```python
from build123d import *

# Parameters (mm, degrees)
CROQUIS1_R                 = 15
SALIENTE_EXTRUIR1_DEPTH    = 175
CROQUIS2_R                 = 4.5
CORTAR_EXTRUIR1_DEPTH      = 177.281025638
CORTAR_EXTRUIR2_START      = 15
CORTAR_EXTRUIR2_DEPTH      = 4
CROQUIS4_R                 = 10
CORTAR_EXTRUIR3_DEPTH      = 177.281025756
CORTAR_EXTRUIR4_DEPTH      = 177.281025756
CORTAR_EXTRUIR4_DEPTH_BACK = 177.281025756
CROQUIS9_R                 = 4.5
CORTAR_EXTRUIR5_START      = 15
CORTAR_EXTRUIR5_DEPTH      = 4
CORTAR_EXTRUIR6_DEPTH      = 177.281025756
CORTAR_EXTRUIR6_DEPTH_BACK = 177.281025756
SALIENTE_EXTRUIR2_START    = 30
CROQUIS16_R                = 17
CROQUIS16_R_2              = 15
SALIENTE_EXTRUIR2_DEPTH    = 30


with BuildPart() as part:
    # Croquis1 → Saliente-Extruir1 (new body)
    with BuildSketch(Plane.XY):
        Circle(CROQUIS1_R)
    extrude(amount=SALIENTE_EXTRUIR1_DEPTH)

    # Croquis2 → Cortar-Extruir1 (cut, symmetric)
    with BuildSketch(Plane(origin=(0, 0, 0), x_dir=(1, 0, 0), z_dir=(0, 1, 0))):
        with Locations(Location((0, -7.5, 0), (0, 0, 270))):
            Circle(CROQUIS2_R)
    cortar_extruir1 = extrude(amount=CORTAR_EXTRUIR1_DEPTH, both=True, mode=Mode.SUBTRACT)

    # Croquis3 → Cortar-Extruir2 (cut)
    with BuildSketch(Plane(origin=(0, 0, 0), x_dir=(1, 0, 0), z_dir=(0, 1, 0)).offset(CORTAR_EXTRUIR2_START)):
        with BuildLine():
            Line((-8.5, -7.5), (-8.5, 0))
            Line((-8.5, 0), (8.5, 0))
            Line((8.5, 0), (8.5, -7.5))
            ThreePointArc((8.5, -7.5), (0, -16), (-8.5, -7.5))
        make_face()
    cortar_extruir2 = extrude(amount=-CORTAR_EXTRUIR2_DEPTH, mode=Mode.SUBTRACT)

    # Croquis4 → Cortar-Extruir3 (cut, symmetric)
    with BuildSketch(Plane(origin=(0, 0, 0), x_dir=(1, 0, 0), z_dir=(0, 1, 0))):
        with Locations((15, 0)):
            Circle(CROQUIS4_R)
    cortar_extruir3 = extrude(amount=CORTAR_EXTRUIR3_DEPTH, both=True, mode=Mode.SUBTRACT)

    # Simetr_a1: Cortar-Extruir1, Cortar-Extruir2, Cortar-Extruir3 across plane
    add(cortar_extruir1.mirror(Plane.XY.offset(87.5)), mode=Mode.SUBTRACT)
    add(cortar_extruir2.mirror(Plane.XY.offset(87.5)), mode=Mode.SUBTRACT)
    add(cortar_extruir3.mirror(Plane.XY.offset(87.5)), mode=Mode.SUBTRACT)

    # Croquis9 → Cortar-Extruir4 (cut, two sides: drawn at the far end of the back side and taken through both)
    with BuildSketch(Plane(origin=(0, 0, 0), x_dir=(1, 0, 0), z_dir=(0, 1, 0)).offset(-CORTAR_EXTRUIR4_DEPTH_BACK)):
        with Locations(Location((0, -79.5, 0), (0, 0, 270))):
            Circle(CROQUIS9_R)
        with Locations(Location((0, -95.5, 0), (0, 0, 270))):
            Circle(CROQUIS9_R)
    extrude(amount=CORTAR_EXTRUIR4_DEPTH + CORTAR_EXTRUIR4_DEPTH_BACK, mode=Mode.SUBTRACT)

    # Croquis10 → Cortar-Extruir5 (cut)
    with BuildSketch(Plane(origin=(0, 0, 0), x_dir=(1, 0, 0), z_dir=(0, 1, 0)).offset(CORTAR_EXTRUIR5_START)):
        with BuildLine():
            Line((8.5, -79.5), (8.5, -95.5))
            ThreePointArc((8.5, -95.5), (0, -104), (-8.5, -95.5))
            Line((-8.5, -95.5), (-8.5, -79.5))
            ThreePointArc((-8.5, -79.5), (0, -71), (8.5, -79.5))
        make_face()
    extrude(amount=-CORTAR_EXTRUIR5_DEPTH, mode=Mode.SUBTRACT)

    # Croquis15 → Cortar-Extruir6 (cut, two sides: drawn at the far end of the back side and taken through both)
    with BuildSketch(Plane(origin=(0, 0, 0), x_dir=(1, 0, 0), z_dir=(0, 1, 0)).offset(-CORTAR_EXTRUIR6_DEPTH_BACK)):
        with BuildLine():
            Line((4, -88), (4, -87))
            ThreePointArc((4, -87), (7.221825407, -79.221825407), (15, -76))
            Line((15, -76), (15, -99))
            ThreePointArc((15, -99), (7.221825407, -95.778174593), (4, -88))
        make_face()
    extrude(amount=CORTAR_EXTRUIR6_DEPTH + CORTAR_EXTRUIR6_DEPTH_BACK, mode=Mode.SUBTRACT)

    # Croquis16 → Saliente-Extruir2 (add)
    with BuildSketch(Plane.XY.offset(SALIENTE_EXTRUIR2_START)):
        Circle(CROQUIS16_R)
        with Locations(Location((0, 0, 0), (0, 0, 124.518107841))):
            Circle(CROQUIS16_R_2, mode=Mode.SUBTRACT)
    saliente_extruir2 = extrude(amount=SALIENTE_EXTRUIR2_DEPTH)

    # Simetr_a2: Saliente-Extruir2 across plane
    add(saliente_extruir2.mirror(Plane.XY.offset(87.5)))


solid = part.part
```
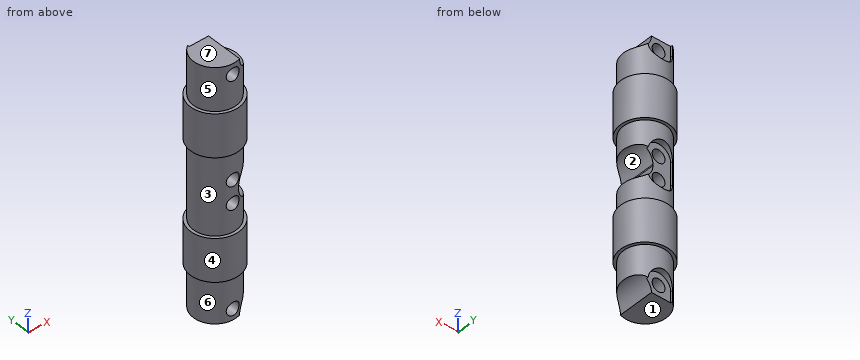
CAD build for the part. Positions are in the model's coordinates, mm. Face numbers are marked on the shaded views. A direction names the side the tool comes from. Round coordinates to 2 decimals unless told otherwise and drop trailing zeros. Order: outer loops, then holes, each group sorted by start corner. A loop starts at its lowest first (then second) coordinate and runs counter-clockwise, first axis right, second up. Notation, with made-up numbers: (89, -25) - (142, -25) arc R16 cw to (142, 3) - close; hole circle Ø1 at (65.5, 72). An arc over 180 degrees is marked (long way). Answer as CSV lines item,"result". Start each with the question number.
1. Saw through at C-C, the plane x = 0. Count the separate pieces of the cut face and the enclosed holes in it, and give its area (3 significant figures).
2. Tool access for the marked faces 5, 6 and 7: list every direction of +Z, -Z, +X, -X, +Y, -Y with a clear straight run to the whole face (end or side of a thin tool).
3. Drill centre lines: L1, parallel to Z at x = 0, y = -7.75; L2, parallel to Z at x = -13.5, y = 8.5; L3, parallel to Z at x = 1.5, y = 0. Where is each one in solid material? Low to high. Write a range as [from, to].
4. Saw through at A-A, the plane z = 93.5. Write the cut outline in (x, y), and give its area (3 significant figures).
5. Pin check, flat tips, straight feed: pin 1 (1.5 mm diameter, centred on x = 6, z = 149.5, fed in from -Y); pin 2 (1 mm diameter, centred on x = 9.5, z = 66.5, fed in from +Y); pin 3 (3 mm diameter, centred on x = -6, z = 120, fed in from -Y); pin 4 (5 mm diameter, centred on x = -0.5, z = 95.5, fed in from +Y). Stop position of each tip, or through.
6. Saw through at B-B, the plane x = 12.5. Write the cut outline in (y, z).
7. Pull direction Z, two halves, no side cores. Call the marked faces 1, 2, 3 and 4: +Z half, -Z half, draft (parallel to the pull), parting line (faces both ways), or undercut.
Model answer:
1,separate pieces,"5"
1,enclosed holes,"0"
1,area,"4,290 mm²"
2,face 5,"+Z"
2,face 6,"-Z"
2,face 7,"+Z, +X, -X, +Y, -Y"
3,L1,"z = [0, 3], [12, 75], [84, 91], [100, 163], [172, 175]"
3,L2,"z = [30, 60], [115, 145]"
3,L3,"z = [0, 3.26], [11.74, 75.26], [83.74, 91.26], [99.74, 163.26], [171.74, 175]"
4,outline,"(-8.5, 11) - (-8.5, 12.36) arc R15 ccw to (-4.03, -14.45) - (-4.03, 11) - close; (4.03, -14.45) arc R15 ccw to (5.47, -13.97) - (5.47, 11) - (4.03, 11) - close"
4,area,"259 mm²"
5,pin 1,"stops at y = -14.05"
5,pin 2,"stops at y = 12"
5,pin 3,"stops at y = -16.39"
5,pin 4,"passes through"
6,outline,"(-11.52, 30) - (-8.29, 30) - (-8.29, 9.68) - (8.29, 9.68) - (8.29, 30) - (11.52, 30) - (11.52, 60) - (8.29, 60) - (8.29, 76.29) - (-8.29, 76.29) - (-8.29, 60) - (-11.52, 60) - close; (-11.52, 115) - (-8.29, 115) - (-8.29, 98.71) - (8.29, 98.71) - (8.29, 115) - (11.52, 115) - (11.52, 145) - (8.29, 145) - (8.29, 165.32) - (-8.29, 165.32) - (-8.29, 145) - (-11.52, 145) - close"
7,face 1,"-Z half"
7,face 2,"undercut"
7,face 3,"undercut"
7,face 4,"draft"
